Build history of the part. All positions in model axes, mm. Face numbers are marked on the shaded views. Give positions to 0.01 mm unless a question says otherwise; leave off trailing zeros. Loops run counter-clockwise (first coordinate to the right, second up) from the corner with the lowest first, then second, coordinate; pieces in that order, holes last. Notation, with made-up numbers: M 79,44 L 90,44 A24 cw 90,71 Z; hole C 1,89.5 d1. An arc over 180 degrees is marked long. Answer as a JSON object with one key per item and string values. Group by question number.
1. Slice it at C-C (y = 6). List the corners of the cut face in (x, z).
2. Slice it at A-A (z = -5.5). List the corners of the cut face in (x, y), then the cut area to 3 significant figures.
3. Slice it at D-D (z = 10.75). List the corners of the cut face in (x, y).
4. Mould opens along X. For the marked faces 1, 2, 3 and 4 say: released by +X, released by -X, zero draft, split by the parting line, or undercut.
5. Slice it at B-B (x = 0.5). List the corners of the cut face in (y, z), then the cut area to 3 significant figures.
6. Drill centre lines: line 1 along Y through (x, z) = (2, -1.75); line 2 along X through (y, z) = (8, 0.5); line 3 along X through (y, z) = (7.75, -7.25). Where is each one in solid material? Low to high. Write a range as [from, to].
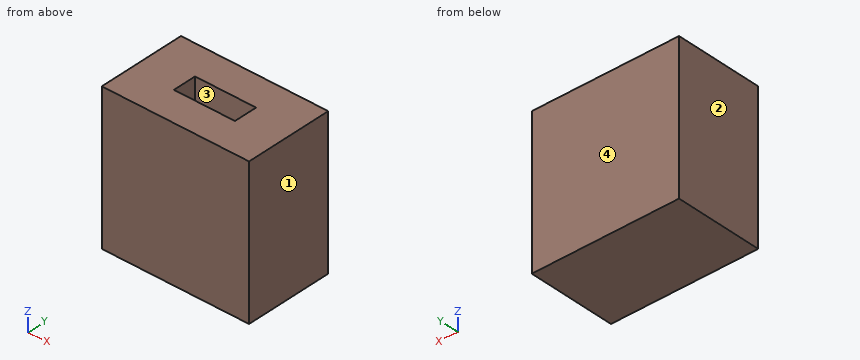
from build123d import *

# Parameters (mm, degrees)
SKETCH1_W           = 25
SKETCH1_H           = 25
BOSS_EXTRUDE1_DEPTH = 15
SKETCH2_W           = 10.366354442
SKETCH2_H           = 4
CUT_EXTRUDE1_DEPTH  = 24
CUT_EXTRUDE1_DRAFT  = -3.5


with BuildPart() as part:
    # Sketch1 → Boss-Extrude1 (new body)
    with BuildSketch(Plane(origin=(0, 0, 0), x_dir=(1, 0, 0), z_dir=(0, 1, 0))):
        Rectangle(SKETCH1_W, SKETCH1_H)
    extrude(amount=BOSS_EXTRUDE1_DEPTH)


with BuildPart() as cut_extrude1_tool:
    # Sketch2 → Cut-Extrude1 (with draft: the straight prism first)
    with BuildSketch(Plane.XY.offset(12.5)):
        with Locations((0, 7.5)):
            Rectangle(SKETCH2_W, SKETCH2_H)
    extrude(amount=-CUT_EXTRUDE1_DEPTH)
    # Cut-Extrude1: the draft: its side faces are tilted about the plane it starts from
    cut_extrude1_sides = [cut_extrude1_tool.faces().sort_by_distance(p)[0] for p in [
        (-5.183177221, 7.5, 0.5),
        (0, 5.5, 0.5),
        (5.183177221, 7.5, 0.5),
        (0, 9.5, 0.5),
    ]]
    draft(cut_extrude1_sides, Plane.XY.offset(12.5), CUT_EXTRUDE1_DRAFT)


with BuildPart() as part_1:
    add(part.part)

    # Cut-Extrude1: cut by cut_extrude1_tool
    add(cut_extrude1_tool.part, mode=Mode.SUBTRACT)


solid = part_1.part
Established:
{
 "1": {"outline": "M -12.5,-12.5 L 12.5,-12.5 L 12.5,12.5 L 5.18,12.5 L 4.68,4.33 L -4.68,4.33 L -5.18,12.5 L -12.5,12.5 Z"},
 "2": {"outline": "M -12.5,0 L 12.5,0 L 12.5,15 L -12.5,15 Z; hole M -4.08,6.6 L 4.08,6.6 L 4.08,8.4 L -4.08,8.4 Z", "area": "360 mm^2"},
 "3": {"outline": "M -12.5,0 L 12.5,0 L 12.5,15 L -12.5,15 Z; hole M -5.08,5.61 L 5.08,5.61 L 5.08,9.39 L -5.08,9.39 Z"},
 "4": {"face 1": "released by +X", "face 2": "released by -X", "face 3": "undercut", "face 4": "zero draft"},
 "5": {"outline": "M 0,-12.5 L 15,-12.5 L 15,12.5 L 9.5,12.5 L 8.03,-11.5 L 6.97,-11.5 L 5.5,12.5 L 0,12.5 Z", "area": "314 mm^2"},
 "6": {"line 1": "y = [0, 6.37], [8.63, 15]", "line 2": "x = [-12.5, -4.45], [4.45, 12.5]", "line 3": "x = [-12.5, -3.98], [3.98, 12.5]"}
}
